Autodesk Inventor part; units mm, degrees
ref_plane "YZ Plane" through (0, 0, 0) normal (1, 0, 0) x (0, 1, 0)
ref_plane "XZ Plane" through (0, 0, 0) normal (0, 1, 0) x (-1, 0, 0)
ref_plane "XY Plane" through (0, 0, 0) normal (0, 0, 1) x (1, 0, 0)
sketch "Sketch1" plane through (0, 0, 0) normal (0, 1, 0) x (-1, 0, 0)
  line L0 (0, -19.05) -> (0, -158.75)
  line L1 (19.05, -177.8) -> (19.05, -177.8)
  line L2 (38.1, -158.75) -> (38.1, -19.05)
  line L3 (19.05, 0) -> (19.05, 0)
  arc A0 (0, -158.75) -> (19.05, -177.8) centre (19.05, -158.75) ccw
  arc A1 (19.05, -177.8) -> (38.1, -158.75) centre (19.05, -158.75) ccw
  arc A2 (38.1, -19.05) -> (19.05, 0) centre (19.05, -19.05) ccw
  arc A3 (19.05, 0) -> (0, -19.05) centre (19.05, -19.05) ccw
  circle A4 centre (19.05, -19.05) radius 3.9688
  circle A5 centre (19.05, -158.75) radius 3.9688
  point P0 (0, 0)
  point P1 (0, -177.8)
  point P2 (38.1, -177.8)
  dimension "d0" = 38.1
  dimension "LengthOfArm_Thiner" = 177.8
  dimension "d2" = 19.05
  dimension "Motor_Shaft_Diameter" = 7.9375
  dimension "d4" = 7.9375
extrude "Extrusion1" add sketch "Sketch1" along normal blind 15.875
sketch "Sketch2" plane through (-38.1, 0, -158.75) normal (-1, 0, 0) x (0, 0, 1)
  line L0 (-19.05, 0) -> (-19.05, 15.875)
  line L1 (-57.15, 4.7625) -> (19.05, 4.7625)
  line L2 (19.05, 4.7625) -> (19.05, 11.1125)
  line L3 (19.05, 11.1125) -> (-57.15, 11.1125)
  line L4 (-57.15, 11.1125) -> (-57.15, 4.7625)
  line L5 (-57.15, 4.7625) -> (19.05, 11.1125) construction
  line L6 (19.05, 4.7625) -> (-57.15, 11.1125) construction
  point P0 (158.75, 0)
  point P1 (-19.05, 7.9375)
  dimension "d7" = 6.35
  dimension "d8" = 38.1
extrude "Extrusion2" cut sketch "Sketch2" against normal up to next
sketch "Sketch3" plane through (0, 15.875, 0) normal (0, 1, 0) x (1, 0, 0)
  circle A0 centre (-19.05, 19.05) radius 3.9687
  line L0 (-24.4521, 26.1937) -> (-13.6479, 26.1937)
  line L1 (-13.6479, 26.1937) -> (-13.6479, 19.8437)
  line L2 (-13.6479, 19.8437) -> (-24.4521, 19.8437)
  line L3 (-24.4521, 19.8437) -> (-24.4521, 26.1937)
  line L4 (-24.4521, 26.1937) -> (-13.6479, 19.8437) construction
  line L5 (-13.6479, 26.1937) -> (-24.4521, 19.8437) construction
  point P0 (0, 0)
  point P1 (-19.05, 23.0187)
  dimension "d11" = 6.35
extrude "Extrusion3" add sketch "Sketch3" against normal up to surface (15.875 mm away) contours L2 A0 | A0 L2 L3 L0 L1 picked at (-18.8857, 21.5143)
properties part number "Arm"
Model file for the job. Use its own axes, mm. A direction names the side the tool comes from. Coordinates: 2 decimals unless noted, no trailing zeros. Loops run counter-clockwise (first coordinate to the right, second up) from the corner with the lowest first, then second, coordinate; pieces in that order, holes last. Notation, with made-up numbers: (-20, -29) -> (-16, -29) arc R23 ccw to (-16, -13) -> close; hole circle Ø1 at (71, 50). An arc over 180 degrees is marked (long way). Answer as a JSON object with one key per item and string values.
Q1. Pull direction X, two halves, no side cores. Call faces 1 (the flat face through (0, 8, -88)), 2 (the cylindrical face through (-19.469, 13.46, -177.795)), 3 (the flat face through (-19, 8, -19.844)), 4 (the flat face through (-19, 0, -88)): released by +X, released by -X, zero draft, split by the parting line, or undercut.
Report:
{"face 1": "released by +X", "face 2": "split by the parting line", "face 3": "undercut", "face 4": "zero draft"}
Q2. 3-axis set-ups, long thin cutter, end or side, ignore diameter. For faces 5 (the cylindrical face through (-22.836, 13.46, -159.942)), 6 (the flat face through (-19, 8, -139.7)): which of +Z, -Z, +X, -X, +Y, -Y reach the whole face in a straight line?
Report:
{"face 5": "+Y, -Y", "face 6": "-Z, +X, -X"}
Q3. Cut at A-A (x = -19.05). List the corners of the cut face in (y, z) (1 decimal), and give its area (3 significant figures).
Report:
{"outline": "(0, -177.8) -> (4.8, -177.8) -> (4.8, -162.7) -> (0, -162.7) -> close; (0, -154.8) -> (4.8, -154.8) -> (4.8, -139.7) -> (11.1, -139.7) -> (11.1, -154.8) -> (15.9, -154.8) -> (15.9, -19.8) -> (0, -19.8) -> close; (0, -15.1) -> (15.9, -15.1) -> (15.9, 0) -> (0, 0) -> close; (11.1, -177.8) -> (15.9, -177.8) -> (15.9, -162.7) -> (11.1, -162.7) -> close", "area": "2,430 mm2"}
Q4. Cut at D-D (x = -27). List the corners of the cut face in (y, z) (1 decimal).
Report:
{"outline": "(0, -176.1) -> (4.8, -176.1) -> (4.8, -139.7) -> (11.1, -139.7) -> (11.1, -176.1) -> (15.9, -176.1) -> (15.9, -1.7) -> (0, -1.7) -> close"}
Q5. Cut at B-B (y = 3.25). List the corners of the cut face in (x, z).
Report:
{"outline": "(-38.1, -158.75) arc R19.05 ccw to (0, -158.75) -> (0, -19.05) arc R19.05 ccw to (-38.1, -19.05) -> close; hole circle Ø7.94 at (-19.05, -158.75); hole (-22.94, -19.84) -> (-15.16, -19.84) arc R3.97 ccw (long way) to start"}
Q6. Cut at C-C (x = -11.5). List the corners of the cut face in (y, z) (1 decimal).
Report:
{"outline": "(0, -176.2) -> (4.8, -176.2) -> (4.8, -139.7) -> (11.1, -139.7) -> (11.1, -176.2) -> (15.9, -176.2) -> (15.9, -1.6) -> (0, -1.6) -> close"}
Q7. Flat gauge pins, fed straight in: P1, Ø6, axis at x = -27, y = 9, coming from the +Z side; P2, Ø7, axis at x = -19.05, z = -158.75, coming from the -Y side; P3, Ø8.5, axis at x = -19, y = 5.5, coming from the +Z side; P4, Ø5, axis at x = -17.5, y = 8, coming from the -Z side. Where does each tip first touch, or does it go through?
Report:
{"P1": "stops at z = -0.65", "P2": "passes through", "P3": "stops at z = 0", "P4": "stops at z = -139.7"}
Q8. Probe probe 1 along Z at (x, y) = (-19.05, 1.85); probe 2 along Y at (x, z) = (-14, -167.5) (1 decimal); probe 3 along Z at (x, y) = (-19.05, 8). List the from-to ranges inside material, lowest first.
Report:
{"probe 1": "z = -177.8 to -162.72, -154.78 to -19.84, -15.08 to 0", "probe 2": "y = 0 to 4.8, 11.1 to 15.9", "probe 3": "z = -139.7 to -19.84, -15.08 to 0"}
